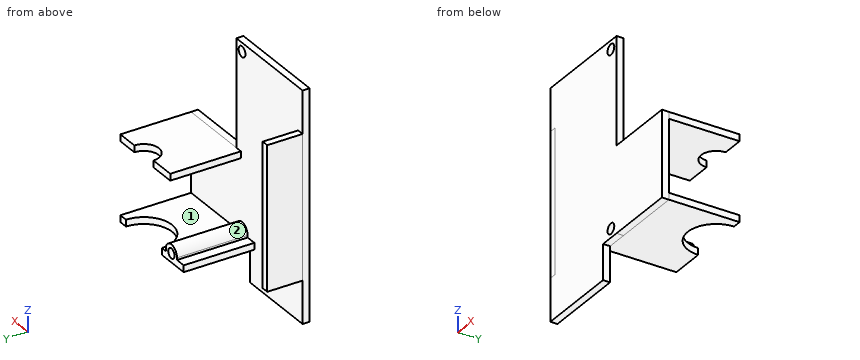
from build123d import *

# Parameters (mm, degrees)
BOSS_EXTRUDE1_DEPTH                 = 2
BOSS_EXTRUDE1_2_DEPTH               = 2
BOSS_EXTRUDE2_DEPTH                 = 1.9
BOSS_EXTRUDE3_DEPTH                 = 1.9
F_16_0MM_DOWEL_HOLE1_D              = 16
F_16_0MM_DOWEL_HOLE1_DEPTH          = 1.9
BOSS_EXTRUDE4_DEPTH                 = 2
F_8_0MM_DOWEL_HOLE1_D               = 8.5
SKETCH10_W                          = 5
SKETCH10_H                          = 3.1
BOSS_EXTRUDE5_DEPTH                 = 20
F_3_0MM_DOWEL_HOLE1_D               = 2.8
F_3_0MM_DOWEL_HOLE1_DEPTH           = 20
F_5_0MM_DOWEL_HOLE1_D               = 3
F_5_0MM_DOWEL_HOLE1_DEPTH           = 2
F_5_0MM_DOWEL_HOLE1_ON_FACE_2_D     = 3
F_5_0MM_DOWEL_HOLE1_ON_FACE_2_DEPTH = 2
FILLET1_RADIUS                      = 2.5
FILLET1_LENGTH                      = 20


with BuildPart() as part:
    # 3DSketch1 → Boss-Extrude1 (new body)
    with BuildSketch(Plane(origin=(0, 0, 0), x_dir=(0.4159263542190885, 0, 0.9093982999027529), z_dir=(0, 1, 0))):
        Polygon((9.774269324, 21.370860048), (0, 0), (58.656190344, -26.827249847), (70.926017793, 0), (43.416719221, 12.581772215), (21.363810448, 22.667986305), (18.868252323, 17.211596506), align=None)
    extrude(amount=BOSS_EXTRUDE1_DEPTH)



with BuildPart() as body_2:
    # 3DSketch1 → Boss-Extrude1 2 (new body)
    with BuildSketch(Plane(origin=(0, 0, 0), x_dir=(0.4159263542190885, 0, 0.9093982999027529), z_dir=(0, 1, 0))):
        Polygon((21.363810448, 22.667986305), (43.416719221, 12.581772215), (51.839227894, 30.997087788), (29.786319121, 41.083301878), align=None)
    extrude(amount=BOSS_EXTRUDE1_2_DEPTH)


with BuildPart() as part_1:
    add(part.part)

    add(body_2.part)  # Boss-Extrude2 merges body 2
    # 3DSketch2 → Boss-Extrude2 (add)
    with BuildSketch(Plane(origin=(27.5, 0, 34.25), x_dir=(0.7110903860866081, 0.7031006064676654, 0), z_dir=(0, 0, 1))):
        Polygon((0, 0), (15.82176109, -15.643988494), (31.289974433, 0), (15.468213342, 15.643988494), align=None)
    extrude(amount=-BOSS_EXTRUDE2_DEPTH)

    # 3DSketch3 → Boss-Extrude3 (add)
    with BuildSketch(Plane(origin=(21.5, 0, 10), x_dir=(0.7889761107100116, 0.6144238738272655, 0), z_dir=(0, 0, -1))):
        Polygon((0, 0), (22.288575128, 17.357474436), (35.805900352, 0), (13.517325224, -17.357474436), align=None)
    extrude(amount=-BOSS_EXTRUDE3_DEPTH)

    # Ø16.0mm Dowel Hole1
    with Locations(Plane(origin=(39.25, 22, 10), x_dir=(-1, 0, 0), z_dir=(0, 0, -1))):
        with Locations((0, 0)):
            Hole(F_16_0MM_DOWEL_HOLE1_D / 2, depth=F_16_0MM_DOWEL_HOLE1_DEPTH)

    # 3DSketch7 → Boss-Extrude4 (add)
    with BuildSketch(Plane(origin=(0, 0, 52.5), x_dir=(0, 0.2840883296913741, -0.9587981127083872), z_dir=(1, 0, 0))):
        Polygon((0, 0), (3.409059956, 11.505577353), (42.240383521, 0), (38.831323565, -11.505577353), align=None)
    extrude(amount=BOSS_EXTRUDE4_DEPTH)

    # Ø8.0mm Dowel Hole1 (through all)
    with Locations(Plane(origin=(39.255, 22, 34.25), x_dir=(1, 0, 0), z_dir=(0, 0, 1))):
        with Locations((0, 0)):
            Hole(F_8_0MM_DOWEL_HOLE1_D / 2)

    # Sketch10 → Boss-Extrude5 (add)
    with BuildSketch(Plane(origin=(0, 2, 0), x_dir=(1, 0, 0), z_dir=(0, 1, 0))):
        with Locations((27, -13.45)):
            Rectangle(SKETCH10_W, SKETCH10_H)
    extrude(amount=BOSS_EXTRUDE5_DEPTH)

    # Ø3.0mm Dowel Hole1
    with Locations(Plane(origin=(27, 22, 12.5), x_dir=(0, 0, 1), z_dir=(0, 1, 0))):
        with Locations((0, 0)):
            Hole(F_3_0MM_DOWEL_HOLE1_D / 2, depth=F_3_0MM_DOWEL_HOLE1_DEPTH)

    # Ø5.0mm Dowel Hole1
    with Locations(Plane(origin=(27, 0, 12.5), x_dir=(0, 0, -1), z_dir=(0, -1, 0))):
        with Locations((0, 0)):
            Hole(F_5_0MM_DOWEL_HOLE1_D / 2, depth=F_5_0MM_DOWEL_HOLE1_DEPTH)

    # Ø5.0mm Dowel Hole1 on face 2
    with Locations(Plane(origin=(27, 2, 62), x_dir=(0, 0, 1), z_dir=(0, 1, 0))):
        with Locations((0, 0)):
            Hole(F_5_0MM_DOWEL_HOLE1_ON_FACE_2_D / 2, depth=F_5_0MM_DOWEL_HOLE1_ON_FACE_2_DEPTH)

    # Fillet1: full round fillet: the end face becomes a half cylinder, R = half its width
    fillet1_face = Plane((27, 12, 15), x_dir=(0, 1, 0), z_dir=(0, 0, 1))  # on the end face: x along it, z out of the body
    fillet1_slab = fillet1_face.offset(-FILLET1_RADIUS / 2) * Box(FILLET1_LENGTH, 2 * FILLET1_RADIUS, FILLET1_RADIUS, mode=Mode.PRIVATE)  # the body's end, R deep
    fillet1_round = Plane((27, 12, 12.5), x_dir=(0, 0, 1), z_dir=(0, 1, 0)) * Cylinder(FILLET1_RADIUS, FILLET1_LENGTH, mode=Mode.PRIVATE)  # its axis R under the face
    add(fillet1_slab - fillet1_round, mode=Mode.SUBTRACT)


solid = part_1.part
Could you check a few things on this model? Use its own coordinates, in mm. Face numbers are marked on the shaded views. A direction names the side the tool comes from. Coordinates: 2 decimals unless noted, no trailing zeros. Write each loop counter-clockwise with the first axis right and the second up, starting at its lowest first coordinate (ties: lowest second). Pieces come first, ordered by that corner, then holes. Notation, with made-up numbers: (-32.5, 6) - (-28.5, 6) arc R15 ccw to (-28.5, 22) - close; hole circle Ø7 at (-13.75, 71.5). An arc over 180 degrees is marked (long way). Put each result on its own line as item: value. Start each with the question number.
Q1. Which directions (+Z, -Z, +X, -X, +Y, -Y) give clear straight access to the entire face, cutting with the end or side of a thin tool? Please do the marked faces 1 and 2.
Q2. I'm going to push flat-ended pins straight in: P1, Ø10, axis at x = 34, y = 14.5, coming from the -Z side; P2, Ø3, axis at y = 7.5, z = 30.5, coming from the +X side; P3, Ø0.7, axis at y = 15, z = 12.5, coming from the -X side; P4, Ø2, axis at x = 27, z = 12.5, coming from the -Y side. Where does each tip first touch, or does it pass through?
Q3. I want a section at D-D on x = 39.25. Write out the boundary of the cut face in (y, z), plus the area to 3 significant figures.
Q4. I want a section at C-C on z = 42. Write out the boundary of the cut face in (x, y).
Q5. Please list where these lines run through material, in increasing order: L1, parallel to X at y = 6.75, z = 12.5; L2, parallel to X at y = 0.55, z = 12.5; L3, parallel to Z at x = 47, y = 14.25.
Q6. I want a section at A-A on y = 13. Write out the boundary of the cut face in (x, z), plus the area to 3 significant figures.
Q7. I want a section at B-B on y = 4.5. Write out the boundary of the cut face in (x, z).
Checks:
1. face 1: +X, +Y
1. face 2: +Y
2. P1: z = 10
2. P2: x = 2
2. P3: x = 24.5
2. P4: through
3. outline: (0, 10) - (14, 10) - (14, 11.9) - (2, 11.9) - (2, 32.35) - (17.75, 32.35) - (17.75, 34.25) - (0, 34.25) - close
3. area: 101 mm²
4. outline: (0, 0) - (29.5, 0) - (29.5, 2) - (2, 2) - (2, 12) - (0, 12) - close
5. L1: 0 to 2, 24.5 to 25.6, 28.4 to 29.5
5. L2: 0 to 25.5, 28.5 to 49.75
5. L3: 10 to 11.9, 32.35 to 34.25
6. outline: (21.5, 10) - (49.75, 10) - (49.75, 11.9) - (29.5, 11.9) - (29.5, 12.5) arc R2.5 ccw to (24.5, 12.5) - (24.5, 11.9) - (21.5, 11.9) - close; (27.5, 32.35) - (49.75, 32.35) - (49.75, 34.25) - (27.5, 34.25) - close; hole circle Ø2.8 at (27, 12.5)
6. area: 103 mm²
7. outline: (0, 12) - (2, 12) - (2, 52.5) - (0, 52.5) - close; (21.5, 10) - (49.75, 10) - (49.75, 11.9) - (29.5, 11.9) - (29.5, 12.5) arc R2.5 ccw to (24.5, 12.5) - (24.5, 11.9) - (21.5, 11.9) - close; (27.5, 32.35) - (49.75, 32.35) - (49.75, 34.25) - (27.5, 34.25) - close; hole circle Ø2.8 at (27, 12.5)
